from build123d import *

# Parameters (mm, degrees)
DOME1_FACE_RADIUS = 3.302
DOME1_HEIGHT      = 2.54
SEEDCUT_DEPTH     = 21.698272826
CIRPATTERN1_COUNT = 8


# Read off the part's stored shape, not the designer's step: Cut-Revolve-Thin3
with BuildPart() as part:
    # Sketch1 → Revolve1 (revolve)
    with BuildSketch(Plane(origin=(0, 0, 0), x_dir=(0, 0, -1), z_dir=(1, 0, 0)), mode=Mode.PRIVATE) as revolve1_sk:
        Polygon((-2.54, 0), (-2.54, 7.493), (0, 7.493), (0, 5.08), (12.7, 5.08), (12.7, 0), align=None)
    revolve(revolve1_sk.sketch.rotate(Axis((0, 0, 9.999244512), (0, 0, -1)), 90), axis=Axis((0, 0, 9.999244512), (0, 0, -1)))

    # Sketch2 → Revolve2 (revolve)
    with BuildSketch(Plane(origin=(0, 0, 0), x_dir=(0, 0, -1), z_dir=(1, 0, 0))):
        with BuildLine():
            Line((-11.531198063, 0), (-2.54, 0))
            Line((-2.54, 0), (-2.54, 6.84268102))
            add(Edge.make_bspline(
                [(-2.54, 6.84268102), (-9.189579749, 6.525332983), (-11.531198063, 0)],
                knots=[0, 0, 0, 1, 1, 1], degree=2))
        make_face()
    revolve(axis=Axis((0, 0, 9.999244512), (0, 0, 1)))

    # Cut-Revolve-Thin3 outline → Cut-Revolve-Thin3 (revolve, cut)
    with BuildSketch(Plane.XZ):
        Polygon((3.302, -10.922), (3.302, -12.7), (5.08, -12.7), (5.08, -6.35), align=None)
    revolve(axis=Axis((0, 0, 0), (0, 0, 1)), mode=Mode.SUBTRACT)

    # Dome1: a dome of height H over a round flat face of radius A is a cap of a sphere of radius (A * A + H * H) / (2 * H)
    dome1_r = (DOME1_FACE_RADIUS * DOME1_FACE_RADIUS + DOME1_HEIGHT * DOME1_HEIGHT) / (2 * DOME1_HEIGHT)
    dome1_base = Plane((0, 0, -12.7), z_dir=(0, 0, -1))
    with Locations(dome1_base.offset(DOME1_HEIGHT - dome1_r)):
        dome1_ball = Sphere(dome1_r, mode=Mode.PRIVATE)
    add(split(dome1_ball, bisect_by=dome1_base, keep=Keep.TOP, mode=Mode.PRIVATE))

    # Sketch4 → SeedCut (cut, through all)
    with BuildSketch(Plane.XY.offset(2.54)):
        with BuildLine():
            Line((0, 7.16784051), (-0.318391894, 7.486232404))
            ThreePointArc((-0.318391894, 7.486232404), (0, 7.493), (0.318391894, 7.486232404))
            Line((0.318391894, 7.486232404), (0, 7.16784051))
        make_face()
    seedcut = extrude(amount=-SEEDCUT_DEPTH, mode=Mode.SUBTRACT)

    # CirPattern1: SeedCut ×8 about axis
    cirpattern1_axis = Axis((0, 0, 0), (0, 0, 1))
    for i in range(1, CIRPATTERN1_COUNT):
        add(seedcut.rotate(cirpattern1_axis, i * 360 / CIRPATTERN1_COUNT), mode=Mode.SUBTRACT)


solid = part.part
Read the model definition and answer for the solid it produces. Units are mm, in the model's axes. A direction names the side the tool comes from. Give positions to 0.01 mm unless a question says otherwise; leave off trailing zeros. Write each loop counter-clockwise with the first axis right and the second up, starting at its lowest first coordinate (ties: lowest second). Pieces come first, ordered by that corner, then holes. Notation, with made-up numbers: M 82.5,11.25 L 131.5,11.25 A11 ccw 131.5,32.25 Z; hole C 69,60 d8. An arc over 180 degrees is marked long. One line per item, written item: value. Start each with the question number.
(1) Find the intervals of material crossed by line 1 (Y direction, x = -1.5, z = -13.5); line 2 (Y direction, x = -1.5, z = 9.75); line 3 (X direction, y = -1.75, z = -2.75), in increasing order.
(2) A tool of negligible diameter and unlimited length cuts with its end or side. For faces 1 (the cylindrical face through (2.83, 6.94, 1.25)), 2 (the flat face through (2, 5, 0)), 3 (the flat face through (-2, -7, 2.54)), from which of +Z, -Z, +X, -X, +Y, -Y can it reach the whole face along a straight path? Write none if from no direction.
(3) Flat-ended cylindrical pins translate along their axes: pin 1 Ø4.5 at (x, y) = (0, -3.5) entering from +Z; pin 2 Ø4 at (x, y) = (3.5, 4.5) entering from +Z; pin 3 Ø1 at (y, z) = (2.5, -5.5) entering from +X. Find the tip coordinate at first contact, or state that the pin passes through.
(4) Find section A-A (z = -8). Determine the outline of the cut face in (x, y), plus the area to 3 significant figures.
Results below:
1. line 1: y = -2.57 to 2.57
1. line 2: y = -2.99 to 2.99
1. line 3: x = -4.77 to 4.77
2. face 1: +Z, -Z, +X, +Y
2. face 2: -Z
2. face 3: +Z
3. pin 1: stops at z = 11.02
3. pin 2: stops at z = 9.46
3. pin 3: stops at x = 4.67
4. outline: C 0,0 d8.88
4. area: 61.9 mm^2
